Source: three-view drawing plus pictorial views. Frame: mm from the lowest corner of the part. Round coordinates to 2 decimals unless told otherwise and drop trailing zeros. Order: outer loops, then holes, each group sorted by start corner. A loop starts at its lowest first (then second) coordinate and runs counter-clockwise, first axis right, second up. Notation, with made-up numbers: (14, 68) -> (43, 68) arc R33 cw to (43, 104) -> close; hole circle Ø8 at (54, 72). An arc over 180 degrees is marked (long way). Answer as CSV lines item,"result".
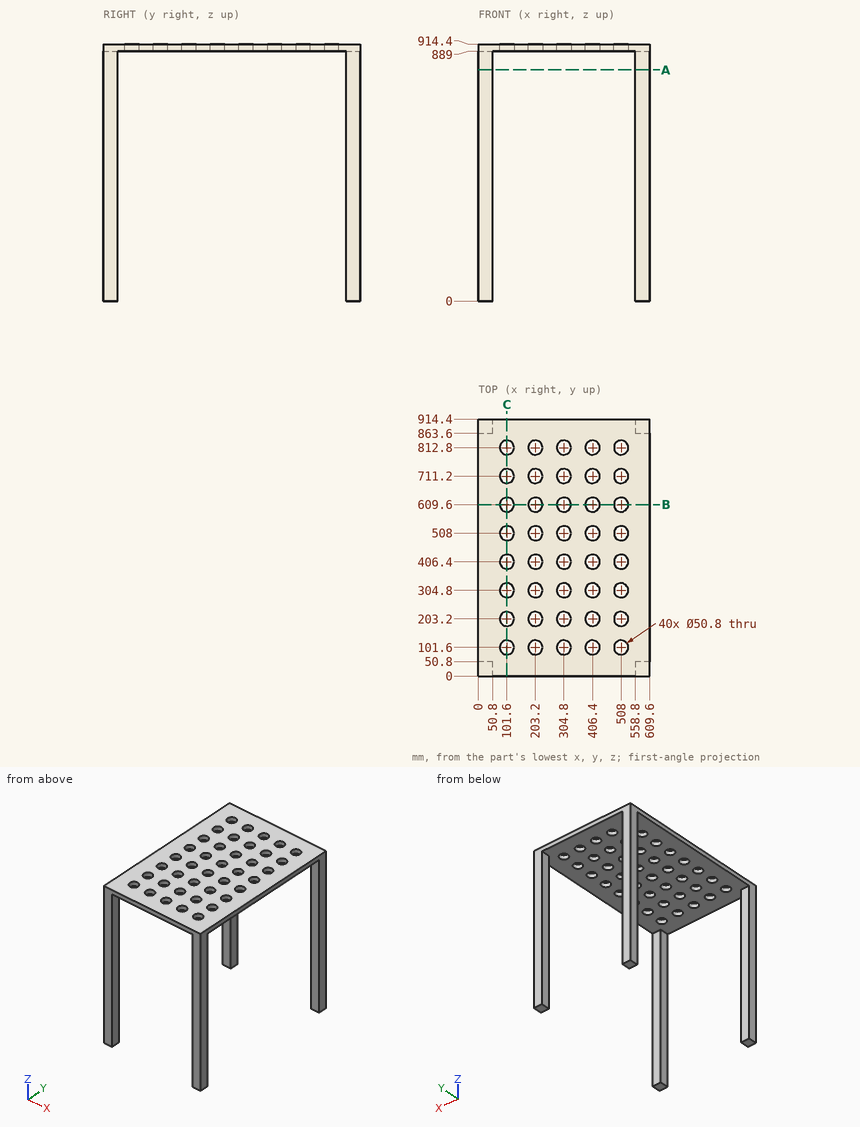
1. Section query C-C on x = 101.6. Give the number of separate pieces and of enclosed holes in the cut face, and give its area (3 significant figures).
Results below:
separate pieces,"9"
enclosed holes,"0"
area,"12,900 mm2"
2. Section query B-B on y = 609.6. Return loops of the section in (x, z).
Results below:
outline,"(0, 889) -> (76.2, 889) -> (76.2, 914.4) -> (0, 914.4) -> close; (127, 889) -> (177.8, 889) -> (177.8, 914.4) -> (127, 914.4) -> close; (228.6, 889) -> (279.4, 889) -> (279.4, 914.4) -> (228.6, 914.4) -> close; (330.2, 889) -> (381, 889) -> (381, 914.4) -> (330.2, 914.4) -> close; (431.8, 889) -> (482.6, 889) -> (482.6, 914.4) -> (431.8, 914.4) -> close; (533.4, 889) -> (609.6, 889) -> (609.6, 914.4) -> (533.4, 914.4) -> close"
3. Pin query (flat end, axial travel): pin 1 (3 mm diameter, centred on x = 225, y = 198.5, fed in from -Z); pin 2 (6 mm diameter, centred on x = 451, y = 746, fed in from -Z). Return the tip coordinate at first contact, or that it passes through.
Results below:
pin 1,"through"
pin 2,"z = 889"
4. Line query: L1, parallel to X at y = 203.2, z = 906.25; L2, parallel to Z at x = 371, y = 543. Output: solid intervals per line, ascending. Write a range as [from, to].
Results below:
L1,"[0, 76.2], [127, 177.8], [228.6, 279.4], [330.2, 381], [431.8, 482.6], [533.4, 609.6]"
L2,"[889, 914.4]"
5. Section query A-A on z = 822. Return loops of the section in (x, y), and give its area (3 significant figures).
Results below:
outline,"(0, 0) -> (50.8, 0) -> (50.8, 50.8) -> (0, 50.8) -> close; (0, 863.6) -> (50.8, 863.6) -> (50.8, 914.4) -> (0, 914.4) -> close; (558.8, 0) -> (609.6, 0) -> (609.6, 50.8) -> (558.8, 50.8) -> close; (558.8, 863.6) -> (609.6, 863.6) -> (609.6, 914.4) -> (558.8, 914.4) -> close"
area,"10,300 mm2"
